from build123d import *

# Parameters (mm, degrees)
SKETCH_3_W          = 20
SKETCH_3_H          = 50
SKETCH_3_R          = 1
SKETCH_3_W_2        = 9
SKETCH_3_H_2        = 21
EXTRUDE_1_DEPTH     = 10
SKETCH_4_R          = 1.7
CUT_EXTRUDE_1_DEPTH = 34.541019662


with BuildPart() as part:
    # 草图3 → 凸台-拉伸1 (new body)
    with BuildSketch(Plane.XY):
        Rectangle(SKETCH_3_W, SKETCH_3_H)
        with Locations((0, -13)):
            Circle(SKETCH_3_R, mode=Mode.SUBTRACT)
        with Locations((0, 12)):
            Circle(SKETCH_3_R, mode=Mode.SUBTRACT)
        Rectangle(SKETCH_3_W_2, SKETCH_3_H_2, mode=Mode.SUBTRACT)
    extrude(amount=EXTRUDE_1_DEPTH)

    # 草图4 → 切除-拉伸1 (cut, through all)
    with BuildSketch(Plane(origin=(10, 0, 0), x_dir=(0, 0, -1), z_dir=(1, 0, 0))):
        with Locations((-5, -20)):
            Circle(SKETCH_4_R)
        with Locations((-5, 20)):
            Circle(SKETCH_4_R)
    extrude(amount=-CUT_EXTRUDE_1_DEPTH, mode=Mode.SUBTRACT)


solid = part.part
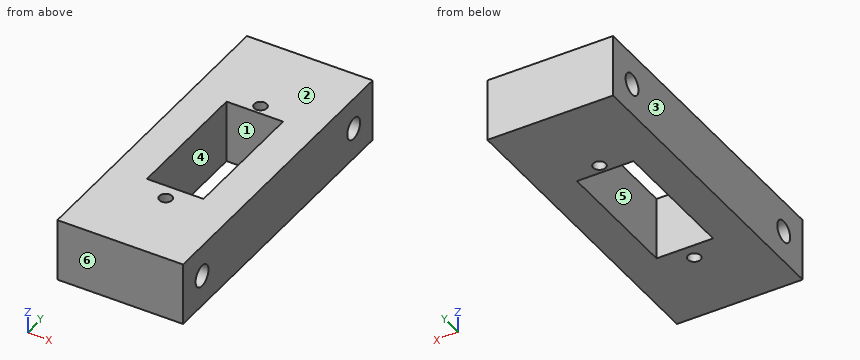
Build history of the part. All positions in model axes, mm. Face numbers are marked on the shaded views. A direction names the side the tool comes from. Coordinates: 2 decimals unless noted, no trailing zeros. Write each loop counter-clockwise with the first axis right and the second up, starting at its lowest first coordinate (ties: lowest second). Pieces come first, ordered by that corner, then holes.
(1) Cut at C-C on z = 8.5. List the corners of the cut face in (x, y).
(2) Drill centre lines: line 1 (Y direction, x = -5, z = 5); line 2 (Y direction, x = 1.5, z = 5); line 3 (Y direction, x = 0, z = 6.75). Where is each one in solid material? Low to high.
(3) 3-axis set-ups, long thin cutter, end or side, ignore diameter. For the marked faces 1 and 2: which of +Z, -Z, +X, -X, +Y, -Y reach the whole face in a straight line?
(4) Mould opens along X. For the marked faces 3, 4, 5 and 6 say: pulls with the +X half, pulls with the -X half, needs draft (parallel to the pull), parting line crosses it, or undercut.
(5) Cut at D-D on y = -1.5. List the corners of the cut face in (x, z).
(6) Cut at A-A on y = 20. List the corners of the cut face in (x, z).
(7) Pin check, flat tip, straight feed: pin 1 Ø1.2 at (x, y) = (0, 12) entering from +Z. Stop position of the tip, or through.
(8) Cut at B-B on z = 5. List the corners of the cut face in (x, y).
Working result:
1. outline: (-10, -25) - (10, -25) - (10, 25) - (-10, 25) - close; hole (-4.5, -10.5) - (4.5, -10.5) - (4.5, 10.5) - (-4.5, 10.5) - close; hole circle Ø2 at (0, -13); hole circle Ø2 at (0, 12)
2. line 1: y = -25 to -21.7, -18.3 to 18.3, 21.7 to 25
2. line 2: y = -25 to -21.7, -18.3 to -10.5, 10.5 to 18.3, 21.7 to 25
2. line 3: y = -25 to -14, -12 to -10.5, 10.5 to 11, 13 to 25
3. face 1: +Z, -Z
3. face 2: +Z, +X, -X, +Y, -Y
4. face 3: pulls with the -X half
4. face 4: undercut
4. face 5: undercut
4. face 6: needs draft
5. outline: (-10, 0) - (-4.5, 0) - (-4.5, 10) - (-10, 10) - close; (4.5, 0) - (10, 0) - (10, 10) - (4.5, 10) - close
6. outline: (-10, 0) - (10, 0) - (10, 3.3) - (-10, 3.3) - close; (-10, 6.7) - (10, 6.7) - (10, 10) - (-10, 10) - close
7. pin 1: passes through
8. outline: (-10, -25) - (10, -25) - (10, -21.7) - (-10, -21.7) - close; (-10, -18.3) - (10, -18.3) - (10, 18.3) - (-10, 18.3) - close; (-10, 21.7) - (10, 21.7) - (10, 25) - (-10, 25) - close; hole (-4.5, -10.5) - (4.5, -10.5) - (4.5, 10.5) - (-4.5, 10.5) - close; hole circle Ø2 at (0, -13); hole circle Ø2 at (0, 12)
